Read the model definition and answer for the solid it produces. Units are mm, in the model's axes. Face numbers are marked on the shaded views. A direction names the side the tool comes from. Round coordinates to 2 decimals unless told otherwise and drop trailing zeros. Order: outer loops, then holes, each group sorted by start corner. A loop starts at its lowest first (then second) coordinate and runs counter-clockwise, first axis right, second up. Notation, with made-up numbers: (-0.75, -34) - (53.25, -34) arc R10 cw to (53.25, -28) - close; hole circle Ø11 at (40, 40.25). An arc over 180 degrees is marked (long way). Put each result on its own line as item: value. Start each with the question number.
Q1. This flat-tipped pin is pushed along its axis until it touches: pin 1 Ø4.5 at (x, y) = (11, -92.5) entering from +Z. Where does it stop, or does it pass through?
Q2. Section A-A on z = 24 is taken. Give the vertices of the cut face in (x, y), then the cut area to 3 significant figures.
Q3. Which of the six approach directions +Z, -Z, +X, -X, +Y, -Y give full straight-line access (tool end or side, diameter ignored) to the marked faces 1 and 2?
Q4. Find the intervals of material crossed by line 1 along Y through (x, z) = (55.5, 33.5); line 2 along Z through (x, y) = (55.5, -93); line 3 along Z through (x, y) = (56.5, -33.5), in increasing order. Write a range as from..to.
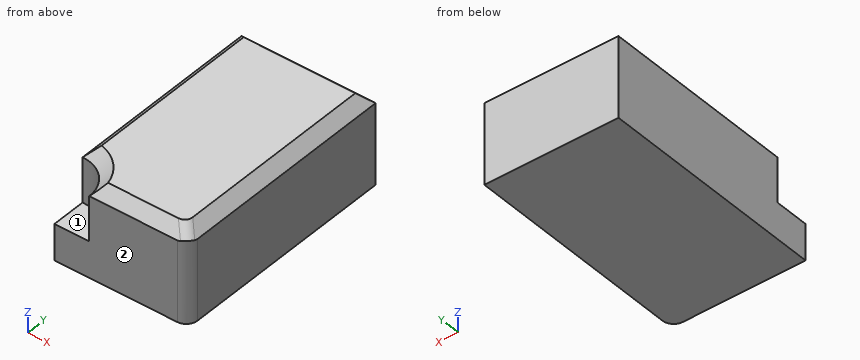
from build123d import *

# Parameters (mm, degrees)
F0_W     = 59.9947497249
F0_H     = 41.1609634757
F1_DEPTH = 103.378
F3_DEPTH = 25
F4_SIZE  = 5
F5_F1_R  = 5
F5_F2_R  = 5


with BuildPart() as f1:
    # F0 (on Front) → F1 (new body)
    with BuildSketch(Plane.XZ):
        with Locations((29.9973748624, 20.5804817379)):
            Rectangle(F0_W, F0_H)
    extrude(amount=F1_DEPTH)

    # F2 (on face) → F3 (cut)
    with BuildSketch(Plane.XY.offset(41.1609634757)):
        with BuildLine():
            ThreePointArc((0, -87.8144259489), (-11.005108751, -114.383108751), (15.5635740511, -103.378))
            Line((15.5635740511, -103.378), (0, -103.378))
            Line((0, -103.378), (0, -87.8144259489))
        make_face()
        with BuildLine():
            Line((0, -103.378), (15.5635740511, -103.378))
            ThreePointArc((15.5635740511, -103.378), (11.005108751, -92.372891249), (0, -87.8144259489))
            Line((0, -87.8144259489), (0, -103.378))
        make_face()
    extrude(amount=-F3_DEPTH, mode=Mode.SUBTRACT)

    # F4
    f4_edges = [f1.edges().sort_by_distance(p)[0] for p in [
        (29.997375, 0, 41.160963),
        (0, -43.907213, 41.160963),
        (11.005109, -92.372891, 41.160963),
        (37.779162, -103.378, 41.160963),
        (59.99475, -51.689, 41.160963),
    ]]
    chamfer(f4_edges, length=F4_SIZE)

    # F5: fillet of radius 5 on 2 edges, made by hand

    # F5_f1
    f5_f1_edges = [f1.edges().sort_by_distance(p)[0] for p in [
        (59.9947497249, -103.378, 18.0804817379),
    ]]
    fillet(f5_f1_edges, radius=F5_F1_R)

    # F5_f2
    f5_f2_edges = [f1.edges().sort_by_distance(p)[0] for p in [
        (56.7625166778, -100.145766953, 39.3931965227),
    ]]
    fillet(f5_f2_edges, radius=F5_F2_R)


solid = f1.part
Findings:
1. pin 1: z = 38.32
2. outline: (0, -87.81) arc R15.56 cw to (15.56, -103.38) - (54.99, -103.38) arc R5 ccw to (59.99, -98.38) - (59.99, 0) - (0, 0) - close
2. area: 6,010 mm2
3. face 1: +Z, -X, -Y
3. face 2: +Z, -Z, +X, -X, -Y
4. line 1: -103.35..0
4. line 2: 0..40.66
4. line 3: 0..39.66
